Work out the finished part from the listing and answer in its coordinate system (mm). A direction names the side the tool comes from. Coordinates: 2 decimals unless noted, no trailing zeros. Write each loop counter-clockwise with the first axis right and the second up, starting at its lowest first coordinate (ties: lowest second). Pieces come first, ordered by that corner, then holes. Notation, with made-up numbers: M 63,-16.5 L 69,-16.5 A29 ccw 69,7.5 Z; hole C -34.75,67 d2. An arc over 180 degrees is marked long. Use CSV: the item, a comma, the result in double quotes.
Autodesk Inventor part; units mm, degrees
ref_plane "YZ Plane" through (0, 0, 0) normal (1, 0, 0) x (0, 1, 0)
ref_plane "XZ Plane" through (0, 0, 0) normal (0, 1, 0) x (-1, 0, 0)
ref_plane "XY Plane" through (0, 0, 0) normal (0, 0, 1) x (1, 0, 0)
sketch "Эскиз1" plane through (0, 0, 0) normal (0, 0, 1) x (1, 0, 0)
  line L0 (-10, 0) -> (10, 0)
  line L1 (-10, 25) -> (-10, 0)
  line L2 (-10, 25) -> (-7, 25)
  line L3 (-7, 25) -> (10, 8)
  line L4 (10, 8) -> (10, 0)
  point P0 (0, 0)
  point P1 (0, 0)
  dimension "d4" = 20
  dimension "d5" = 25
  dimension "d6" = 3
  dimension "d7" = 135
extrude "Выдавливание1" add sketch "Эскиз1" along normal mid plane 45
sketch "Эскиз3" plane through (-7, 25, -22.5) normal (0.7071, 0.7071, 0) x (-0.7071, 0.7071, 0)
  line L0 (-4.5208, 40) -> (-19.5208, 40)
  line L1 (-19.5208, 40) -> (-19.5208, 16.8)
  line L2 (-19.5208, 16.8) -> (-4.5208, 16.8)
  line L3 (-4.5208, 16.8) -> (-4.5208, 40)
  line L4 (-24.0416, 45) -> (0, 45)
  line L5 (-5.0208, 11.8) -> (-19.0208, 11.8)
  line L6 (-19.0208, 11.8) -> (-19.0208, 3.5)
  line L7 (-19.0208, 3.5) -> (-5.0208, 3.5)
  line L8 (-5.0208, 3.5) -> (-5.0208, 11.8)
  line L9 (0, 0) -> (-24.0416, 0)
  point P0 (-22.6274, 22.5)
  point P1 (-12.0208, 11.8)
  point P2 (-12.0208, 16.8)
  point P3 (-12.0208, 3.5)
  point P4 (-12.0208, 0)
  dimension "d8" = 23.2
  dimension "d9" = 15
  dimension "d10" = 5
  dimension "d11" = 14
  dimension "d12" = 8.3
  dimension "d13" = 5
extrude "Выдавливание2" cut sketch "Эскиз3" against normal blind 10
sketch "Эскиз7" plane through (0, 0, 22.5) normal (0, 0, 1) x (1, 0, 0)
  line L0 (10, 0) -> (-10, 0)
  line L1 (0, 8.1005) -> (-10, 18.1005)
  line L2 (10, 8) -> (-7, 25)
  line L3 (6.8033, 11.1967) -> (-3.8033, 21.8033)
  line L4 (10, 8) -> (10, 0)
  line L5 (-7, 25) -> (10, 8)
  line L6 (-7, 25) -> (10, 8)
  line L7 (0, 8.1005) -> (0, 2)
  line L8 (0, 2) -> (-10, 2)
  line L9 (-10, 2) -> (-10, 0)
  line L10 (-10, 0) -> (10, 0)
  line L11 (10, 8) -> (10, 0)
  line L12 (-10, 18.1005) -> (-10, 22)
  line L13 (-10, 22) -> (-7, 25)
  line L14 (-10, 25) -> (-10, 0)
  point P0 (0, 0)
  point P1 (1.5, 16.5)
  dimension "d22" = 7
  dimension "d24" = 2
  dimension "d25" = 10
  dimension "d26" = 135
extrude "Выдавливание4" cut sketch "Эскиз7" against normal through all contours L0 L9 L8 L7 L1 L12 L13 L2 L4 keep common part
sketch "Эскиз8" plane through (0, 0, -22.5) normal (0, 0, -1) x (-1, 0, 0)
  line L0 (10, 2) -> (0, 2)
  line L1 (-10, 0) -> (10, 0)
  line L2 (10, 2) -> (-10, 2)
  line L3 (-10, 2) -> (-10, 0)
  line L4 (-10, 0) -> (10, 0)
  line L5 (10, 0) -> (10, 2)
  point P0 (0, 0)
extrude "Выдавливание5" add sketch "Эскиз8" along normal blind 10
chamfer "Фаска1" distance 5 angle 45 2 edges at (10, 1, -32.5) (-10, 1, -32.5)
mirror "Зеркальное отражение1" about plane through (0, 0, 0) normal (0, 0, 1) of "Выдавливание5", "Фаска1"
sketch "Эскиз9" plane through (0, 2, 22.5) normal (0, 1, 0) x (1, 0, 0)
  line L0 (10, 0) -> (-7, 0)
  line L1 (0, 0) -> (0, 45)
  point P0 (0, 22.5)
  point P1 (0, 50)
  point P2 (0, -5)
  point P3 (0, 22.5)
  dimension "d41" = 55
  dimension "d42" = 5
hole "Отверстие1" at (0, 2, -27.5) at (0, 2, 27.5) direction (0, -1, 0) diameter 3.2 end through all
properties part number "Indicator"
Item 1: The part is cut by section C-C (y = 15.25). Write down the section's boundary in (x, z), then the cut area to 3 significant figures.
Answer:
outline,"M -7.15,-22.5 L 2.75,-22.5 L 2.75,-19 L -7.15,-19 Z; M -7.15,-10.7 L 2.75,-10.7 L 2.75,-5.7 L -7.15,-5.7 Z; M -7.15,17.5 L 2.75,17.5 L 2.75,22.5 L -7.15,22.5 Z"
area,"134 mm2"
Item 2: The part is cut by section A-A (z = -14). Write down the section's boundary in (x, y).
Answer:
outline,"M -10,0 L 10,0 L 10,8 L 6.45,11.55 L 0,5.1 L 0,2 L -10,2 Z; M -10,18.1 L -8.4,16.5 L -3.45,21.45 L -7,25 L -10,22 Z"
Item 3: A tool of negligible diameter and unlimited length cuts with its end or side. For faces 1 (the face through (-9.4, 17.5, 0.3)), 2 (the face through (0, 11, -22.5)), 3 (the face through (3.3, 8.4, -14.8)), 4 (the face through (-1, 14, 17.5)), 5 (the face through (-5.9, 19, -14.9)), from which of +Z, -Z, +X, -X, +Y, -Y can it reach the whole face along a straight path? Write none if from no direction.
Answer:
face 1,"+Z, -Z, -X"
face 2,"-Z, +X, -X, +Y"
face 3,"-X, +Y"
face 4,"none"
face 5,"+X"
Item 4: The part is cut by section B-B (x = -5.75). Write down the section's boundary in (y, z).
Answer:
outline,"M 0,-31.75 L 2,-31.75 L 2,31.75 L 0,31.75 Z; M 13.85,-22.5 L 23.75,-22.5 L 23.75,22.5 L 13.85,22.5 L 13.85,17.5 L 19.86,17.5 L 19.86,-5.7 L 13.85,-5.7 L 13.85,-10.7 L 19.15,-10.7 L 19.15,-19 L 13.85,-19 Z"
Item 5: The part is cut by section D-D (z = -3). Write down the section's boundary in (x, y), then the cut area to 3 significant figures.
Answer:
outline,"M -10,0 L 10,0 L 10,8 L 6.8,11.2 L 0,4.39 L 0,2 L -10,2 Z; M -10,18.1 L -8.75,16.85 L -3.8,21.8 L -7,25 L -10,22 Z"
area,"132 mm2"
Item 6: Given pin 1 (1.9 mm diameter, centred on x = 0, z = 27.5, fed in from -Y); pin 2 (6 mm diameter, centred on x = 3, z = 10.5, fed in from +Y); pin 3 (2 mm diameter, centred on x = -4, z = 9, fed in from +Y); pin 4 (4.5 mm diameter, centred on x = -4, y = 9.5, fed in from +Z), each flat-ended and moving along its own axis, determine where each tip first touches the part or whether it passes through.
Answer:
pin 1,"passes through"
pin 2,"stops at y = 10.39"
pin 3,"stops at y = 23"
pin 4,"stops at z = 22.5"
Item 7: Consider probe 1 along Z at (x, y) = (0, 1.65); probe 2 along X at (y, z) = (0.45, -27.5); probe 3 along Z at (x, y) = (4.5, 12). Determine where each line is inside the solid, lowest interval first.
Answer:
probe 1,"z = -32.5 to -29.1, -25.9 to 25.9, 29.1 to 32.5"
probe 2,"x = -10 to -1.6, 1.6 to 10"
probe 3,"z = -22.5 to -19, -10.7 to -5.7, 17.5 to 22.5"
Item 8: For a pull along X with two mould halves and no side action, classify faces 6 (the face through (-1.08, 0.99, -28.68)), 7 (the face through (-4, 22, 0)), 8 (the face through (0, 4, 0)), 9 (the face through (-1, 14, -19)) as released by +X, released by -X, zero draft, split by the parting line, or undercut.
Answer:
face 6,"undercut"
face 7,"released by +X"
face 8,"released by -X"
face 9,"zero draft"
